```python
from build123d import *

# Parameters (mm, degrees)
SKETCH1_R           = 12
SKETCH1_R_2         = 1.75
BOSS_EXTRUDE1_DEPTH = 8


with BuildPart() as part:
    # Sketch1 → Boss-Extrude1 (new body)
    with BuildSketch(Plane.XY):
        with BuildLine():
            Line((36.15, 21.15), (-36.15, 21.15))
            Line((-36.15, 21.15), (-36.15, -57))
            Line((-36.15, -57), (-36.15, -65))
            Line((-36.15, -65), (-16.15, -65))
            Line((-16.15, -65), (-16.15, -50))
            Line((-16.15, -50), (-3.25, -50))
            ThreePointArc((-3.25, -50), (-3.108578644, -49.941421356), (-3.05, -49.8))
            Line((-3.05, -49.8), (-3.05, -36.2))
            ThreePointArc((-3.05, -36.2), (-3.108578644, -36.058578644), (-3.25, -36))
            Line((-3.25, -36), (-4.8, -36))
            ThreePointArc((-4.8, -36), (-4.941421356, -35.941421356), (-5, -35.8))
            Line((-5, -35.8), (-5, -31))
            ThreePointArc((-5, -31), (-4.941421356, -30.858578644), (-4.8, -30.8))
            Line((-4.8, -30.8), (-3.25, -30.8))
            ThreePointArc((-3.25, -30.8), (-3.108578644, -30.741421356), (-3.05, -30.6))
            Line((-3.05, -30.6), (-3.05, -24.8))
            ThreePointArc((-3.05, -24.8), (-2.464213562, -23.385786438), (-1.05, -22.8))
            Line((-1.05, -22.8), (1.05, -22.8))
            ThreePointArc((1.05, -22.8), (2.464213562, -23.385786438), (3.05, -24.8))
            Line((3.05, -24.8), (3.05, -30.6))
            ThreePointArc((3.05, -30.6), (3.108578644, -30.741421356), (3.25, -30.8))
            Line((3.25, -30.8), (4.8, -30.8))
            ThreePointArc((4.8, -30.8), (4.941421356, -30.858578644), (5, -31))
            Line((5, -31), (5, -35.8))
            ThreePointArc((5, -35.8), (4.941421356, -35.941421356), (4.8, -36))
            Line((4.8, -36), (3.25, -36))
            ThreePointArc((3.25, -36), (3.108578644, -36.058578644), (3.05, -36.2))
            Line((3.05, -36.2), (3.05, -49.8))
            ThreePointArc((3.05, -49.8), (3.108578644, -49.941421356), (3.25, -50))
            Line((3.25, -50), (16.15, -50))
            Line((16.15, -50), (16.15, -65))
            Line((16.15, -65), (36.15, -65))
            Line((36.15, -65), (36.15, -57))
            Line((36.15, -57), (36.15, 21.15))
        make_face()
        Circle(SKETCH1_R, mode=Mode.SUBTRACT)
        with Locations((-15.5, 15.5)):
            Circle(SKETCH1_R_2, mode=Mode.SUBTRACT)
        with Locations((15.5, 15.5)):
            Circle(SKETCH1_R_2, mode=Mode.SUBTRACT)
        with Locations((15.5, -15.5)):
            Circle(SKETCH1_R_2, mode=Mode.SUBTRACT)
        with Locations((-15.5, -15.5)):
            Circle(SKETCH1_R_2, mode=Mode.SUBTRACT)
    extrude(amount=BOSS_EXTRUDE1_DEPTH)


solid = part.part
```
Work out the finished part from the listing and answer in its coordinate system (mm). A direction names the side the tool comes from. Coordinates: 2 decimals unless noted, no trailing zeros. Loops run counter-clockwise (first coordinate to the right, second up) from the corner with the lowest first, then second, coordinate; pieces in that order, holes last. Notation, with made-up numbers: (79.25, -4) - (96.25, -4) arc R10 cw to (96.25, 0) - close; hole circle Ø4 at (67.5, 81.25). An arc over 180 degrees is marked (long way). Use a Markdown table: item, result.
Item 1: Find section A-A, the plane y = -15.5. Determine the outline of the cut face in (x, z).
Evaluation:
| item | result |
|---|---|
| outline | (-36.15, 0) - (-17.25, 0) - (-17.25, 8) - (-36.15, 8) - close; (-13.75, 0) - (13.75, 0) - (13.75, 8) - (-13.75, 8) - close; (17.25, 0) - (36.15, 0) - (36.15, 8) - (17.25, 8) - close |
Item 2: Find section B-B, the plane x = 0. Determine the outline of the cut face in (y, z).
Evaluation:
| item | result |
|---|---|
| outline | (-22.8, 0) - (-12, 0) - (-12, 8) - (-22.8, 8) - close; (12, 0) - (21.15, 0) - (21.15, 8) - (12, 8) - close |
Item 3: For faces 4 (the flat face through (5, -33, 4)), 5 (the flat face through (10, -50, 4)), 6 (the flat face through (36.15, -23, 4)), determine the directions among +Z, -Z, +X, -X, +Y, -Y from which every point of the face is accessible in a straight line to the end or side of a thin tool.
Evaluation:
| item | result |
|---|---|
| face 4 | +Z, -Z |
| face 5 | +Z, -Z, -Y |
| face 6 | +Z, -Z, +X, +Y, -Y |
Item 4: The mould has two halves that part along Y. Classify faces 1 (the cylindrical face through (-14.6, 17, 3.9)), 2 (the flat face through (-26, -65, 4)), 3 (the flat face through (3.05, -28, 4)): +Y half, -Y half, draft (parallel to the pull), parting line (faces both ways), or undercut.
Evaluation:
| item | result |
|---|---|
| face 1 | undercut |
| face 2 | -Y half |
| face 3 | draft |
Item 5: Find section D-D, the plane z = 4.5. State how many separate pieces and enclosed holes the cut face has, and give its area (3 significant figures).
Evaluation:
| item | result |
|---|---|
| separate pieces | 1 |
| enclosed holes | 5 |
| area | 5,070 mm2 |
Item 6: Consider probe 1 along Y at (x, z) = (15.5, 4.75); probe 2 along X at (y, z) = (-36.5, 2.5); probe 3 along Y at (x, z) = (3.5, 7.5). Determine where each line is inside the solid, lowest interval first. Write a range as from..to.
Evaluation:
| item | result |
|---|---|
| probe 1 | y = -50..-17.25, -13.75..13.75, 17.25..21.15 |
| probe 2 | x = -36.15..-3.05, 3.05..36.15 |
| probe 3 | y = -50..-36, -30.8..-11.48, 11.48..21.15 |
Item 7: Given pin 1 Ø2 at (x, z) = (0.5, 1.5) entering from -Y; pin 2 Ø2.5 at (x, z) = (12, 6) entering from -Y; pin 3 Ø3 at (x, y) = (15.5, 15.5) entering from -Z; pin 4 Ø1 at (x, z) = (0, 3) entering from -Y, each flat-ended and moving along its own axis, determine where each tip first touches the part or whether it passes through.
Evaluation:
| item | result |
|---|---|
| pin 1 | stops at y = -22.85 |
| pin 2 | stops at y = -50 |
| pin 3 | passes through |
| pin 4 | stops at y = -22.8 |
Item 8: Find section C-C, the plane y = -41. Determine the outline of the cut face in (x, z).
Evaluation:
| item | result |
|---|---|
| outline | (-36.15, 0) - (-3.05, 0) - (-3.05, 8) - (-36.15, 8) - close; (3.05, 0) - (36.15, 0) - (36.15, 8) - (3.05, 8) - close |
